Here's how the part is built. I have some questions about the finished solid (model axes, mm). Face numbers are marked on the shaded views. A direction names the side the tool comes from. Round coordinates to 2 decimals unless told otherwise and drop trailing zeros. Write each loop counter-clockwise with the first axis right and the second up, starting at its lowest first coordinate (ties: lowest second). Pieces come first, ordered by that corner, then holes. Notation, with made-up numbers: (16, 14) -> (23, 14) arc R3 cw to (23, 18) -> close; hole circle Ø6 at (8, 66). An arc over 180 degrees is marked (long way). Answer as CSV lines item,"result".
```python
from build123d import *

# Parameters (mm, degrees)
BOSS_EXTRUDE1_DEPTH = 3
SKETCH2_R           = 1.95
CUT_EXTRUDE1_DEPTH  = 25.703238654
SKETCH3_W           = 3
SKETCH3_H           = 4
CUT_EXTRUDE2_DEPTH  = 25.703238654
SKETCH4_W           = 3
SKETCH4_H           = 16
CUT_EXTRUDE3_DEPTH  = 10


with BuildPart() as part:
    # Sketch1 → Boss-Extrude1 (new body)
    with BuildSketch(Plane.XY):
        Polygon((8.5, -20), (5.5, -20), (5.5, -23), (2.5, -23), (2.5, -20), (-2.5, -20), (-2.5, -23), (-5.5, -23), (-5.5, -20), (-8.5, -20), (-8.5, 20), (8.5, 20), align=None)
    extrude(amount=BOSS_EXTRUDE1_DEPTH)

    # Sketch2 → Cut-Extrude1 (cut, through all)
    with BuildSketch(Plane.XY.offset(3)):
        with Locations((-4.25, 16)):
            Circle(SKETCH2_R)
        with Locations((4.25, 16)):
            Circle(SKETCH2_R)
    extrude(amount=-CUT_EXTRUDE1_DEPTH, mode=Mode.SUBTRACT)

    # Sketch3 → Cut-Extrude2 (cut, through all)
    with BuildSketch(Plane.XY.offset(3)):
        with Locations((-7, -18)):
            Rectangle(SKETCH3_W, SKETCH3_H)
        with Locations((7, -18)):
            Rectangle(SKETCH3_W, SKETCH3_H)
    extrude(amount=-CUT_EXTRUDE2_DEPTH, mode=Mode.SUBTRACT)

    # Sketch4 → Cut-Extrude3 (cut)
    with BuildSketch(Plane.XY.offset(3)):
        with Locations((-7, -8)):
            Rectangle(SKETCH4_W, SKETCH4_H)
        with Locations((7, -8)):
            Rectangle(SKETCH4_W, SKETCH4_H)
    extrude(amount=-CUT_EXTRUDE3_DEPTH, mode=Mode.SUBTRACT)


solid = part.part
```
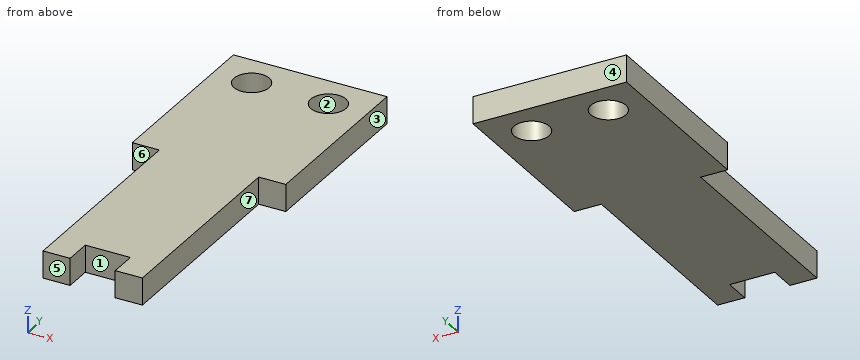
1. If I drill on line 1 (Y direction, x = 4.25, z = 1.35); line 2 (X direction, y = -6, z = 2.75); line 3 (Y direction, x = 0, z = 1.7), over which ranges is the centre line in solid material (lowest first)?
Numbers:
line 1,"y = -23 to 14.05, 17.95 to 20"
line 2,"x = -5.5 to 5.5"
line 3,"y = -20 to 20"
2. Suppose I cut it at D-D on y = -19. Please give me the cut outline in (x, z), and give its area (3 significant figures).
Numbers:
outline,"(-5.5, 0) -> (5.5, 0) -> (5.5, 3) -> (-5.5, 3) -> close"
area,"33.0 mm^2"
3. If we mould it in two halves opening along X, with no side actions, what happens to the marked faces 1, 2, 3 and 4? For each: released by +X, released by -X, zero draft, split by the parting line, or undercut.
Numbers:
face 1,"undercut"
face 2,"undercut"
face 3,"released by +X"
face 4,"zero draft"
4. For pin 1 Ø1.5 at (y, z) = (-7.5, 1.5) entering from -X; pin 2 Ø10 at (x, y) = (1, -18) entering from -Z; pin 3 Ø1.5 at (y, z) = (-21.5, 2) entering from +X; pin 4 Ø0.9 at (x, z) = (6.5, 1) entering from -Y, each with a flat end and sliding along its axis, tell me the tip position at first contact or that it passes through.
Numbers:
pin 1,"stops at x = -5.5"
pin 2,"stops at z = 0"
pin 3,"stops at x = 5.5"
pin 4,"stops at y = 0"
5. Suppose I cut it at B-B on z = 0.65. Please give me the cut outline in (x, y), and give its area (3 significant figures).
Numbers:
outline,"(-8.5, 0) -> (-5.5, 0) -> (-5.5, -23) -> (-2.5, -23) -> (-2.5, -20) -> (2.5, -20) -> (2.5, -23) -> (5.5, -23) -> (5.5, 0) -> (8.5, 0) -> (8.5, 20) -> (-8.5, 20) -> close; hole circle Ø3.9 at (-4.25, 16); hole circle Ø3.9 at (4.25, 16)"
area,"554 mm^2"
6. On a 3-axis mill with a long thin cutter (end or side, diameter ignored), from which of +Z, -Z, +X, -X, +Y, -Y can I reach the whole of each face in a straight line? I mean the marked faces 5, 6 and 7. Say none if no direction works.
Numbers:
face 5,"+Z, -Z, +X, -X, -Y"
face 6,"+Z, -Z, -X, -Y"
face 7,"+Z, -Z, +X, -Y"
7. Suppose I cut it at A-A on y = 16. Please give me the cut outline in (x, z), and give its area (3 significant figures).
Numbers:
outline,"(-8.5, 0) -> (-6.2, 0) -> (-6.2, 3) -> (-8.5, 3) -> close; (-2.3, 0) -> (2.3, 0) -> (2.3, 3) -> (-2.3, 3) -> close; (6.2, 0) -> (8.5, 0) -> (8.5, 3) -> (6.2, 3) -> close"
area,"27.6 mm^2"
8. Suppose I cut it at C-C on x = 4.25. Please give me the cut outline in (y, z).
Numbers:
outline,"(-23, 0) -> (14.05, 0) -> (14.05, 3) -> (-23, 3) -> close; (17.95, 0) -> (20, 0) -> (20, 3) -> (17.95, 3) -> close"
